The listing builds one solid part. Answer for the finished solid, in the listing's coordinates (mm). A direction names the side the tool comes from. Give positions to 0.01 mm unless a question says otherwise; leave off trailing zeros. Loops run counter-clockwise (first coordinate to the right, second up) from the corner with the lowest first, then second, coordinate; pieces in that order, holes last. Notation, with made-up numbers: (48.5, 17.25) - (81.5, 17.25) arc R22 ccw to (81.5, 47.25) - close; hole circle Ø4 at (73, 65). An arc over 180 degrees is marked (long way). One line per item, written item: value. Start each with the question number.
from build123d import *

# Parameters (mm, degrees)
F0_W     = 2.5
F0_H     = 8
F1_DEPTH = 24.25
F2_W     = 8
F2_H     = 3
F3_DEPTH = 7


with BuildPart() as f1:
    # F0 (on Front) → F1 (new body, symmetric)
    with BuildSketch(Plane.XZ):
        Polygon((-12.75, 12.5), (-12.75, 8), (-10.25, 8), (10.25, 8), (12.75, 8), (12.75, 12.5), align=None)
        with Locations((-11.5, 4)):
            Rectangle(F0_W, F0_H)
        with Locations((11.5, 4)):
            Rectangle(F0_W, F0_H)
    extrude(amount=F1_DEPTH, both=True)

    # F2 (on face) → F3 (cut)
    with BuildSketch(Plane.XZ.offset(24.25)):
        with Locations((0, 11)):
            Rectangle(F2_W, F2_H)
    extrude(amount=-F3_DEPTH, mode=Mode.SUBTRACT)


solid = f1.part
1. A cutting plane is placed at C-C (z = 11). Determine the outline of the cut face in (x, y), plus the area to 3 significant figures.
2. A cutting plane is placed at D-D (x = 9). Determine the outline of the cut face in (y, z).
3. For faces 1 (the flat face through (0, -24.25, 9)), 2 (the flat face through (0, 0, 8)), 3 (the flat face through (-4, -21, 11)), determine the directions among +Z, -Z, +X, -X, +Y, -Y from which every point of the face is accessible in a straight line to the end or side of a thin tool.
4. A cutting plane is placed at B-B (y = 9.5). Determine the outline of the cut face in (x, z).
5. A cutting plane is placed at A-A (z = 7). Determine the outline of the cut face in (x, y), plus the area to 4 significant figures.
6. Find the intervals of material crossed by L1, parallel to X at y = -18, z = 7.75; L2, parallel to Z at x = -8.25, y = -3; L3, parallel to Z at x = 1.25, y = -21, in increasing order. Write a range as [from, to].
7. Flat-ended cylindrical pins translate along their axes: pin 1 (6 mm diameter, centred on x = 3.5, y = 2, fed in from -Z); pin 2 (0.9 mm diameter, centred on x = -0.5, z = 11.5, fed in from -Y); pin 3 (6 mm diameter, centred on x = -4, z = 3.5, fed in from -Y); pin 4 (2 mm diameter, centred on x = -1, y = -22, fed in from +Z). Find the tip coordinate at first contact, or state that the pin passes through.
Results below:
1. outline: (-12.75, -24.25) - (-4, -24.25) - (-4, -17.25) - (4, -17.25) - (4, -24.25) - (12.75, -24.25) - (12.75, 24.25) - (-12.75, 24.25) - close
1. area: 1,180 mm^2
2. outline: (-24.25, 8) - (24.25, 8) - (24.25, 12.5) - (-24.25, 12.5) - close
3. face 1: +Z, -Z, +X, -X, -Y
3. face 2: -Z, +Y, -Y
3. face 3: +Z, -Y
4. outline: (-12.75, 0) - (-10.25, 0) - (-10.25, 8) - (10.25, 8) - (10.25, 0) - (12.75, 0) - (12.75, 12.5) - (-12.75, 12.5) - close
5. outline: (-12.75, -24.25) - (-10.25, -24.25) - (-10.25, 24.25) - (-12.75, 24.25) - close; (10.25, -24.25) - (12.75, -24.25) - (12.75, 24.25) - (10.25, 24.25) - close
5. area: 242.5 mm^2
6. L1: x = [-12.75, -10.25], [10.25, 12.75]
6. L2: z = [8, 12.5]
6. L3: z = [8, 9.5]
7. pin 1: stops at z = 8
7. pin 2: stops at y = -17.25
7. pin 3: passes through
7. pin 4: stops at z = 9.5
